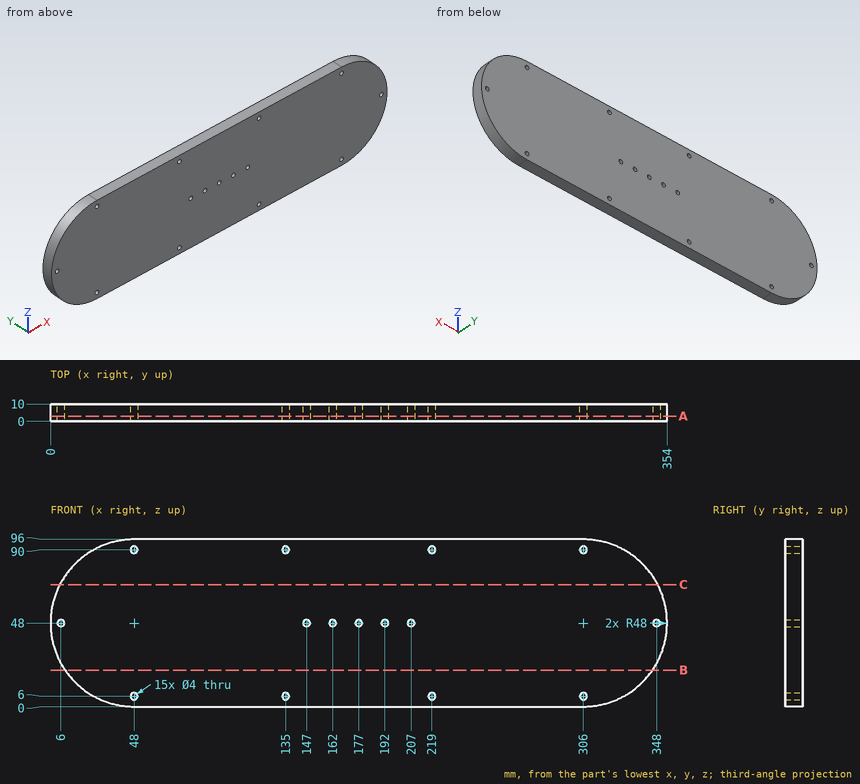
Design review of the part shown in the three views and the two pictorial views. Dimensions are in mm from the part's minimum x, y and z. Give positions to 0.01 mm unless a question says otherwise; leave off trailing zeros. Write each loop counter-clockwise with the first axis right and the second up, starting at its lowest first coordinate (ties: lowest second). Pieces come first, ordered by that corner, then holes. Notation, with made-up numbers: M 4.5,43 L 32.5,43 A22 ccw 32.5,71 Z; hole C 2.25,-11 d3. An arc over 180 degrees is marked long. Answer as CSV lines item,"result".
1. Consider section B-B, the plane z = 21. Write out the cut boundary in (x, y).
Findings:
outline,"M 8.31,0 L 345.69,0 L 345.69,10 L 8.31,10 Z"
2. For pin 1 (6 mm diameter, centred on x = 316.5, z = 23, fed in from -Y); pin 2 (6 mm diameter, centred on y = 3.5, z = 16, fed in from +X); pin 3 (5 mm diameter, centred on y = 4, z = 15.5, fed in from -X); pin 4 (2 mm diameter, centred on y = 3.5, z = 86, fed in from +X), all flat-tipped, find the tip position at first contact; note any pin that passes through.
Findings:
pin 1,"stops at y = 0"
pin 2,"stops at x = 344.25"
pin 3,"stops at x = 10.53"
pin 4,"stops at x = 336.58"
3. Consider section A-A, the plane y = 3. Count the separate pieces of the cut face and the enclosed holes in it, then the cut area to 3 significant figures.
Findings:
separate pieces,"1"
enclosed holes,"15"
area,"31,800 mm2"
4. Wall thickness on line 1 (Z direction, x = 219, y = 7.5); line 2 (Z direction, x = 207, y = 5); line 3 (X direction, y = 3.75, z = 80): over which ranges is each line inside the solid? List them lowest first.
Findings:
line 1,"z = 0 to 4, 8 to 88, 92 to 96"
line 2,"z = 0 to 46, 50 to 96"
line 3,"x = 12.22 to 341.78"
5. Consider section C-C, the plane z = 70. Write out the cut boundary in (x, y), then the cut area to 3 significant figures.
Findings:
outline,"M 5.34,0 L 348.66,0 L 348.66,10 L 5.34,10 Z"
area,"3,430 mm2"
